Read the model definition and answer for the solid it produces. Units are mm, in the model's axes. A direction names the side the tool comes from. Give positions to 0.01 mm unless a question says otherwise; leave off trailing zeros. Loops run counter-clockwise (first coordinate to the right, second up) from the corner with the lowest first, then second, coordinate; pieces in that order, holes last.
(1) Each of these flat-tipped pins is pushed along its axis until it touches: P1, Ø4, axis at x = -59, y = -1, coming from the -Z side; P2, Ø1.1, axis at x = -44.5, y = 18.5, coming from the +Z side. Where does it stop, or does it pass through?
(2) Straight lines are drawn through the part: probe 1 along Y at (x, z) = (-4, 23); probe 2 along Y at (x, z) = (24, 12.75). For each, find the intervals that lie inside material, in ascending order.
(3) Find section B-B, the plane z = 8. Write down the section's boundary in (x, y), then the cut area to 3 significant figures.
(4) Find section A-A, the plane x = -2. Write down the section's boundary in (y, z).
(5) Which of the six approach directions +Z, -Z, +X, -X, +Y, -Y give full straight-line access (tool end or side, diameter ignored) to faces 4 (the face through (0, 40.5, 10)), 5 (the face through (-3, -42, 19.4)), 6 (the face through (60, 2, 25))?
(6) Determine the mould class of faces 1 (the face through (140, -2, 12)), 2 (the face through (-33, 33, 0)), 3 (the face through (32.831, -32.613, 9.564)) for opening direction X: pulls with the +X half, pulls with the -X half, needs draft (parallel to the pull), parting line crosses it, or undercut.
```python
from build123d import *

# Parameters (mm, degrees)
F0_W     = 280
F0_H     = 280
F1_DEPTH = 25
F2_W     = 6.5
F2_H     = 5.5
F2_W_2   = 11
F2_H_2   = 6.5
F3_DEPTH = 2.5
F4_W     = 87.6
F4_H     = 87.6
F5_DEPTH = 5.6


with BuildPart() as f1:
    # F0 (on Top) → F1 (new body)
    with BuildSketch(Plane.XY):
        Rectangle(F0_W, F0_H)
        Polygon((-40.5, 24.943651), (-24.943651, 40.5), (24.943651, 40.5), (40.5, 24.943651), (40.5, -24.943651), (24.943651, -40.5), (-24.943651, -40.5), (-40.5, -24.943651), align=None, mode=Mode.SUBTRACT)
    extrude(amount=F1_DEPTH)

    # F2 (on face) → F3 (cut)
    with BuildSketch(Plane.XY.offset(25)):
        with Locations((-20, 43.25)):
            Rectangle(F2_W, F2_H)
        with Locations((-20, 37.75)):
            Rectangle(F2_W, F2_H)
        with Locations((20, 43.25)):
            Rectangle(F2_W, F2_H)
        with Locations((20, 37.75)):
            Rectangle(F2_W, F2_H)
        with Locations((-40.5, 20)):
            Rectangle(F2_W_2, F2_H_2)
        with Locations((-40.5, -20)):
            Rectangle(F2_W_2, F2_H_2)
    extrude(amount=-F3_DEPTH, mode=Mode.SUBTRACT)

    # F4 (on face) → F5 (cut)
    with BuildSketch(Plane.XY.offset(25)):
        Rectangle(F4_W, F4_H)
    extrude(amount=-F5_DEPTH, mode=Mode.SUBTRACT)


solid = f1.part
```
Entries:
1. P1: stops at z = 0
1. P2: stops at z = 22.5
2. probe 1: y = -140 to -43.8, 43.8 to 140
2. probe 2: y = -140 to -40.5, 40.5 to 140
3. outline: (-140, -140) - (140, -140) - (140, 140) - (-140, 140) - close; hole (-40.5, -24.94) - (-24.94, -40.5) - (24.94, -40.5) - (40.5, -24.94) - (40.5, 24.94) - (24.94, 40.5) - (-24.94, 40.5) - (-40.5, 24.94) - close
3. area: 72,300 mm2
4. outline: (-140, 0) - (-40.5, 0) - (-40.5, 19.4) - (-43.8, 19.4) - (-43.8, 25) - (-140, 25) - close; (40.5, 0) - (140, 0) - (140, 25) - (43.8, 25) - (43.8, 19.4) - (40.5, 19.4) - close
5. face 4: +Z, -Z
5. face 5: +Z
5. face 6: +Z, +X, -X, +Y, -Y
6. face 1: pulls with the +X half
6. face 2: needs draft
6. face 3: undercut
